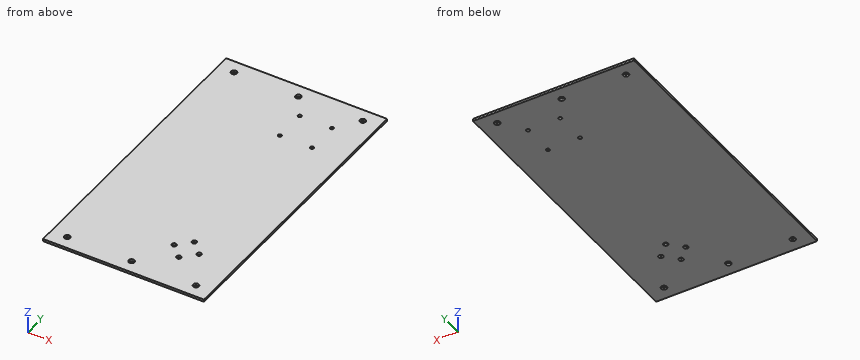
from build123d import *

# Parameters (mm, degrees)
SKETCH1_W            = 155
SKETCH1_H            = 285.39
BOSS_EXTRUDE1_DEPTH  = 2.305
M5_CLEARANCE_HOLE1_D = 5.5
SKETCH4_R            = 2.25
SKETCH4_R_2          = 1.7
CUT_EXTRUDE1_DEPTH   = 3.305


with BuildPart() as part:
    # Sketch1 → Boss-Extrude1 (new body)
    with BuildSketch(Plane.XY):
        Rectangle(SKETCH1_W, SKETCH1_H)
    extrude(amount=BOSS_EXTRUDE1_DEPTH)

    # M5 Clearance Hole1 (through all)
    with Locations(Plane.XY.offset(2.305)):
        with Locations((-62, 129.995), (0, 129.995), (-62, -129.995), (0, -129.995), (62, -129.995)):
            m5_clearance_hole1 = Hole(M5_CLEARANCE_HOLE1_D / 2)

    # Sketch4 → Cut-Extrude1 (cut, through all)
    with BuildSketch(Plane.XY.offset(2.305)):
        with Locations((30.1, -81)):
            Circle(SKETCH4_R)
        with Locations((42.1, -93)):
            Circle(SKETCH4_R)
        with Locations((30.1, -105)):
            Circle(SKETCH4_R)
        with Locations((18.1, -93)):
            Circle(SKETCH4_R)
        with Locations((45.6, 108.5)):
            Circle(SKETCH4_R_2)
        with Locations((14.6, 77.5)):
            Circle(SKETCH4_R_2)
        with Locations((45.6, 77.5)):
            Circle(SKETCH4_R_2)
        with Locations((14.6, 108.5)):
            Circle(SKETCH4_R_2)
    extrude(amount=-CUT_EXTRUDE1_DEPTH, mode=Mode.SUBTRACT)

    # Mirror1: M5 Clearance Hole1 across plane
    add(m5_clearance_hole1.mirror(Plane.ZX), mode=Mode.SUBTRACT)


solid = part.part
Model file for the job. Use its own axes, mm. Give positions to 0.01 mm unless a question says otherwise; leave off trailing zeros. Order: outer loops, then holes, each group sorted by start corner. A loop starts at its lowest first (then second) coordinate and runs counter-clockwise, first axis right, second up. Notation, with made-up numbers: (44.25, 45) - (52.25, 45) arc R14 cw to (52.25, 53) - close; hole circle Ø6 at (-18, 19). An arc over 180 degrees is marked (long way). Return JSON: item names as keys, results as strings.
1) Flat gauge pin, fed straight in: P1, Ø7, axis at x = 0, y = -129.995, coming from the -Z side. Where does the tip first touch, or does it go through?
Geometry says:
{"P1": "z = 0"}
2) Probe line 1 (X direction, y = -130, z = 0.85); line 2 (X direction, y = 108.5, z = 1.45); line 3 (Y direction, x = 45.6, z = 0.55) (3 decimals). List the from-to ranges inside material, lowest first. Write a range as from..to.
Geometry says:
{"line 1": "-77.5..-64.75, -59.25..-2.75, 2.75..59.25, 64.75..77.5", "line 2": "-77.5..12.9, 16.3..43.9, 47.3..77.5", "line 3": "-142.695..75.8, 79.2..106.8, 110.2..142.695"}
3) Cut at A-A, the plane x = 0. Give the cut face in (y, z) (3 decimals).
Geometry says:
{"outline": "(-142.695, 0) - (-132.745, 0) - (-132.745, 2.305) - (-142.695, 2.305) - close; (-127.245, 0) - (127.245, 0) - (127.245, 2.305) - (-127.245, 2.305) - close; (132.745, 0) - (142.695, 0) - (142.695, 2.305) - (132.745, 2.305) - close"}
